```python
from build123d import *

# Parameters (mm, degrees)
F0_W     = 101.6
F0_H     = 50.8
F1_DEPTH = 50.8
F2_R     = 6.35
F3_DEPTH = 50.801
F4_W     = 12.7
F4_H     = 25.4
F6_W     = 19.9219
F6_H     = 6.35


with BuildPart() as f1:
    # F0 (on Top) → F1 (new body)
    with BuildSketch(Plane.XY):
        with Locations((-0.469463, -0.556229)):
            Rectangle(F0_W, F0_H)
    extrude(amount=F1_DEPTH)

    # F2 (on face) → F3 (cut, through all)
    with BuildSketch(Plane.XY.offset(50.8)):
        with Locations((-38.569463, 12.143771)):
            Circle(F2_R)
        with Locations((37.630537, 12.143771)):
            Circle(F2_R)
        with Locations((37.630537, -13.256229)):
            Circle(F2_R)
        with Locations((-38.569463, -13.256229)):
            Circle(F2_R)
    extrude(amount=-F3_DEPTH, mode=Mode.SUBTRACT)

    # F4 (on Front) → F5 (revolve)
    with BuildSketch(Plane.XZ):
        with Locations((-6.35, 63.5)):
            Rectangle(F4_W, F4_H)
    revolve(axis=Axis((0, 0, 63.5), (0, 0, -1)))

    # F6 (on Front) → F7 (revolve, cut)
    with BuildSketch(Plane.XZ):
        with Locations((-17.58095, 60.325)):
            Rectangle(F6_W, F6_H)
    revolve(axis=Axis((0, 0, 76.2), (0, 0, -1)), mode=Mode.SUBTRACT)


solid = f1.part
```
Source: CAD feature listing. Evaluate the final solid. Frame: model axes, mm. A direction names the side the tool comes from. Give positions to 0.01 mm unless a question says otherwise; leave off trailing zeros. Write each loop counter-clockwise with the first axis right and the second up, starting at its lowest first coordinate (ties: lowest second). Pieces come first, ordered by that corner, then holes. Notation, with made-up numbers: (79.5, -32.5) - (100.5, -32.5) arc R20 cw to (100.5, -18.5) - close; hole circle Ø10 at (52, 3). An arc over 180 degrees is marked (long way). One line per item, written item: value. Start each with the question number.
Q1. Material intervals for probe 1 along X at (y, z) = (-13, 34.5); probe 2 along X at (y, z) = (17.5, 28); probe 3 along Z at (x, y) = (30.5, -4), sorted ascending. Write a range as from..to.
Q2. Draft query along Z for faces 1 (the face through (-12, 5, 50.8)), 2 (the face through (1.65, -7.44, 60.37)), 3 (the face through (-5.5, -5.5, 63.5)), 4 (the face through (2.75, -12.4, 54.02)). Return one class per face: +Z half, -Z half, draft (parallel to the pull), parting line (faces both ways), or undercut.
Q3. Section query A-A, the plane z = 35. Return the cut outline in (x, y), then the cut area to 3 significant figures.
Q4. First-contact query: pin 1 Ø2 at (x, y) = (15, -11.5) entering from +Z; pin 2 Ø4 at (x, z) = (-6.5, 53.5) entering from -Y; pin 3 Ø7.5 at (x, y) = (37.63, 12.14) entering from +Z; pin 4 Ø1.5 at (x, z) = (5, 56) entering from +Y. Flat tips, straight axial feed; report the tip coordinate or a pass-through.
Q5. Set-up query: faces 5 (the face through (-5.5, -5.5, 57.15)), 6 (the face through (2.75, -12.4, 69.94)), 7 (the face through (-32.513, 14.051, 25.756)). Return all of +Z, -Z, +X, -X, +Y, -Y with unobstructed straight access to the full face (end or side cutting, diameter ignored); none if empty.
Q6. Section query B-B, the plane x = 0. Return the cut outline in (y, z).
Q7. Section query C-C, the plane y = 0. Return the cut outline in (x, z).
Q8. Section query D-D, the plane z = 69. Return the cut outline in (x, y).
Answer:
1. probe 1: x = -51.27..-44.91, -32.22..31.29, 43.98..50.33
1. probe 2: x = -51.27..-41.98, -35.16..34.22, 41.04..50.33
1. probe 3: z = 0..50.8
2. face 1: +Z half
2. face 2: undercut
2. face 3: undercut
2. face 4: draft
3. outline: (-51.27, -25.96) - (50.33, -25.96) - (50.33, 24.84) - (-51.27, 24.84) - close; hole circle Ø12.7 at (-38.57, -13.26); hole circle Ø12.7 at (-38.57, 12.14); hole circle Ø12.7 at (37.63, -13.26); hole circle Ø12.7 at (37.63, 12.14)
3. area: 4,650 mm2
4. pin 1: stops at z = 50.8
4. pin 2: stops at y = -11.88
4. pin 3: passes through
4. pin 4: stops at y = 11.97
5. face 5: none
5. face 6: +Z
5. face 7: +Z, -Z
6. outline: (-25.96, 0) - (24.84, 0) - (24.84, 50.8) - (12.7, 50.8) - (12.7, 57.15) - (7.62, 57.15) - (7.62, 63.5) - (12.7, 63.5) - (12.7, 76.2) - (-12.7, 76.2) - (-12.7, 63.5) - (-7.62, 63.5) - (-7.62, 57.15) - (-12.7, 57.15) - (-12.7, 50.8) - (-25.96, 50.8) - close
7. outline: (-51.27, 0) - (50.33, 0) - (50.33, 50.8) - (12.7, 50.8) - (12.7, 57.15) - (7.62, 57.15) - (7.62, 63.5) - (12.7, 63.5) - (12.7, 76.2) - (-12.7, 76.2) - (-12.7, 63.5) - (-7.62, 63.5) - (-7.62, 57.15) - (-12.7, 57.15) - (-12.7, 50.8) - (-51.27, 50.8) - close
8. outline: circle Ø25.4 at (0, 0)
